from build123d import *

# Parameters (mm, degrees)
F1_DEPTH      = 63.5
F1_DEPTH_BACK = 1.0668
F2_W          = 2.54
F2_H          = 17.78
F3_DEPTH      = 2.54
F4_DEPTH      = 2.54
F5_R          = 1.77830971


# Not quite as in the source:
# - a feature names something its author has since deleted; it is built from what else it names


with BuildPart() as f1:
    # F0 (on Right) → F1 (new body, two sides)
    with BuildSketch(Plane.YZ) as f1_sk:
        Polygon((2.9329393675, 0), (0, 5.08), (-2.9329393675, 0), align=None)
    extrude(amount=F1_DEPTH)
    extrude(f1_sk.sketch, amount=-F1_DEPTH_BACK)

    # F2 (on Front) → F3 (join, symmetric)
    with BuildSketch(Plane.XZ):
        with Locations((21.7847247761, 8.89)):
            Rectangle(F2_W, F2_H)
    extrude(amount=F3_DEPTH, both=True)

    # F2 (on Front) → F4 (join, symmetric)
    with BuildSketch(Plane.XZ):
        Polygon((-9.746064432, 17.78), (0, 0), (0, 4.6337883681), (-7.206064432, 17.78), align=None)
    extrude(amount=F4_DEPTH, both=True)

    # F5
    f5_edges = [f1.edges().sort_by_distance(p)[0] for p in [
        (-1.0668, 0, 0),
    ]]
    fillet(f5_edges, radius=F5_R)


solid = f1.part
Source: CAD feature listing. Evaluate the final solid. Frame: model axes, mm. A direction names the side the tool comes from. Coordinates: 2 decimals unless noted, no trailing zeros. Loops run counter-clockwise (first coordinate to the right, second up) from the corner with the lowest first, then second, coordinate; pieces in that order, holes last. Notation, with made-up numbers: (14, 52) -> (48, 52) arc R12 ccw to (48, 71) -> close; hole circle Ø1 at (37, -11.75). An arc over 180 degrees is marked (long way). Answer in a Markdown table with one row per item. Add a question column.
Q1. Section C-C on x = 55. Return the cut outline in (y, z), and give its area (3 significant figures).
Q2. Reachability of faces 1 (the face through (-0.56, 0.041, 0.535)), 2 (the face through (0, -2, 4)), 3 (the face through (0, 2, 4)), 4 (the face through (22, 2.54, 9)), 5 (the face through (22, -2.54, 9)) from +Z, -Z, +X, -X, +Y, -Y: full face, straight path, thin tool, end or side. Return the list, or none.
Q3. Section B-B on y = -1.2. Return the cut outline in (x, z), and give its area (3 significant figures).
Q4. Section A-A on z = 15.75. Return the cut outline in (x, y), and give its area (3 significant figures).
Q5. Contact query for flat-ended pins moving along their axis: pin 1 Ø0.8 at (x, z) = (21.5, 8) entering from -Y; pin 2 Ø2 at (x, z) = (21.5, 9.5) entering from +Y; pin 3 Ø0.7 at (y, z) = (2, 2.5) entering from +X. Output: stop coordinate, or through.
Q6. Ray query, line 1 along X through (y, z) = (1.9, 3.5); line 2 along X through (y, z) = (-0.35, 5); line 3 along Z through (x, y) = (38.5, 1.8). Return the intervals inside material, ascending.
Computed values:
| question | item | result |
|---|---|---|
| 1 | outline | (-2.93, 0) -> (2.93, 0) -> (0, 5.08) -> close |
| 1 | area | 14.9 mm^2 |
| 2 | face 1 | -Z, -X, +Y, -Y |
| 2 | face 2 | +Z, -Y |
| 2 | face 3 | +Z, +Y |
| 2 | face 4 | +Z, +X, -X, +Y |
| 2 | face 5 | +Z, +X, -X, -Y |
| 3 | outline | (-9.75, 17.78) -> (-1.07, 1.95) -> (-1.07, 1.78) arc R1.78 ccw to (0.71, 0) -> (63.5, 0) -> (63.5, 3) -> (23.05, 3) -> (23.05, 17.78) -> (20.51, 17.78) -> (20.51, 3) -> (0, 3) -> (0, 4.63) -> (-7.21, 17.78) -> close |
| 3 | area | 268 mm^2 |
| 4 | outline | (-8.63, -2.54) -> (-6.09, -2.54) -> (-6.09, 2.54) -> (-8.63, 2.54) -> close; (20.51, -2.54) -> (23.05, -2.54) -> (23.05, 2.54) -> (20.51, 2.54) -> close |
| 4 | area | 25.8 mm^2 |
| 5 | pin 1 | stops at y = -2.54 |
| 5 | pin 2 | stops at y = 2.54 |
| 5 | pin 3 | stops at x = 23.05 |
| 6 | line 1 | x = -1.92 to 0, 20.51 to 23.05 |
| 6 | line 2 | x = -2.74 to -0.2, 20.51 to 23.05 |
| 6 | line 3 | z = 0 to 1.96 |
